The listing builds one solid part. Answer for the finished solid, in the listing's coordinates (mm). Round coordinates to 2 decimals unless told otherwise and drop trailing zeros. Loops run counter-clockwise (first coordinate to the right, second up) from the corner with the lowest first, then second, coordinate; pieces in that order, holes last. Notation, with made-up numbers: (-4.75, 73) -> (30.25, 73) arc R19 ccw to (30.25, 91) -> close; hole circle Ø3 at (11, -10.75). An arc over 180 degrees is marked (long way). Write each question's results on one line, items separated by ' | '. Start each with the question number.
(1) Flat-ended cylindrical pins translate along their axes: pin 1 (1.5 mm diameter, centred on y = 4.5, z = -3.5, fed in from +X); pin 2 (4 mm diameter, centred on x = 0.5, y = 4, fed in from +Z); pin 3 (0.8 mm diameter, centred on y = 4, z = -5, fed in from +X). Find the tip coordinate at first contact, or state that the pin passes through.
(2) The part is cut by section C-C (z = 1.25). Determine the outline of the cut face in (x, y) (3 decimals).
(3) The part is cut by section A-A (x = -0.5). Determine the outline of the cut face in (y, z).
(4) The part is cut by section B-B (y = 2.25). Determine the outline of the cut face in (x, z), plus the area to 4 significant figures.
Autodesk Inventor part; units mm, degrees
ref_plane "YZ Plane" through (0, 0, 0) normal (1, 0, 0) x (0, 1, 0)
ref_plane "XZ Plane" through (0, 0, 0) normal (0, 1, 0) x (-1, 0, 0)
ref_plane "XY Plane" through (0, 0, 0) normal (0, 0, 1) x (1, 0, 0)
sketch "Sketch1" plane through (0, 0, 0) normal (0, 1, 0) x (-1, 0, 0)
  line L0 (-6.425, -4.45) -> (6.425, -4.45)
  line L1 (6.425, -4.45) -> (6.425, 4.45)
  line L2 (6.425, 4.45) -> (-6.425, 4.45)
  line L3 (-6.425, 4.45) -> (-6.425, -4.45)
  line L4 (-6.425, -4.45) -> (6.425, 4.45) construction
  line L5 (6.425, -4.45) -> (-6.425, 4.45) construction
  line L6 (-2.3625, -4.45) -> (2.3625, -4.45)
  line L7 (2.3625, -4.45) -> (2.3625, -14)
  line L8 (-2.3625, -14) -> (-2.3625, -4.45)
  line L9 (1.45, -15.01) -> (-1.45, -15.01)
  line L10 (2.3625, -14) -> (1.45, -15.01)
  line L11 (-1.45, -15.01) -> (-2.3625, -14)
extrude "Extrusion1" add sketch "Sketch1" along normal blind 0.1
sketch "Sketch2" plane through (0, 0, 0) normal (0, -1, 0) x (1, 0, 0)
  line L0 (-2.3625, -4.45) -> (2.3625, -4.45)
  line L1 (-2.3625, -5.45) -> (2.3625, -5.45)
  point P0 (0, 0)
  dimension "d2" = 1
bend part "Bend Part1" radius 1 angle 90 line through (-2.3625, 0, -4.45) along (1, 0, 0) centre toward (0, 1, 0) moving side (0, 0, -1) both sides no
properties part number "ECoG64Ch"
Checked values:
1) pin 1: passes through | pin 2: stops at z = -5.35 | pin 3: stops at x = 2.36
2) outline: (-6.425, 0) -> (6.425, 0) -> (6.425, 0.1) -> (-6.425, 0.1) -> close
3) outline: (0, -4.45) arc R1 ccw to (1, -5.45) -> (9.99, -5.45) -> (9.99, -5.35) -> (1, -5.35) arc R0.9 cw to (0.1, -4.45) -> (0.1, 4.45) -> (0, 4.45) -> close
4) outline: (-2.36, -5.45) -> (2.36, -5.45) -> (2.36, -5.35) -> (-2.36, -5.35) -> close | area: 0.4725 mm2
